The listing builds one solid part. Answer for the finished solid, in the listing's coordinates (mm). Face numbers are marked on the shaded views. A direction names the side the tool comes from. Round coordinates to 2 decimals unless told otherwise and drop trailing zeros. Loops run counter-clockwise (first coordinate to the right, second up) from the corner with the lowest first, then second, coordinate; pieces in that order, holes last. Notation, with made-up numbers: (5.5, 64) -> (43.5, 64) arc R17 cw to (43.5, 78) -> close; hole circle Ø2 at (-12, -19.75). An arc over 180 degrees is marked (long way). One line per question, with ' | ' between items.
from build123d import *

# Parameters (mm, degrees)
F0_W     = 50.8
F0_H     = 50.8
F1_DEPTH = 7.62
F2_T     = -1.27
F3_R     = 1.27
F4_DEPTH = 25.4


with BuildPart() as f1:
    # F0 (on Top) → F1 (new body)
    with BuildSketch(Plane.XY):
        with Locations((25.4, 25.4)):
            Rectangle(F0_W, F0_H)
    extrude(amount=F1_DEPTH)

    # F2
    f2_openings = [f1.faces().sort_by_distance(p)[0] for p in [
        (25.4, 25.4, 7.62),
    ]]
    offset(amount=F2_T, openings=f2_openings)

    # F3 (on face) → F4 (cut)
    with BuildSketch(Plane.XY.offset(1.27)):
        with Locations((3.81, 18.601548)):
            Circle(F3_R)
    extrude(amount=-F4_DEPTH, mode=Mode.SUBTRACT)


solid = f1.part
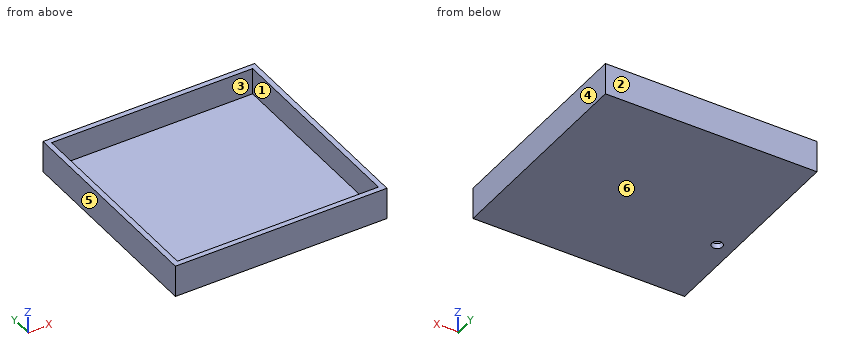
Q1. A cutting plane is placed at C-C on y = 45. Give the vertices of the cut face in (x, z).
Numbers:
outline: (0, 0) -> (50.8, 0) -> (50.8, 7.62) -> (49.53, 7.62) -> (49.53, 1.27) -> (1.27, 1.27) -> (1.27, 7.62) -> (0, 7.62) -> close
Q2. A cutting plane is placed at B-B on z = 6.75. Give the vertices of the cut face in (x, y).
Numbers:
outline: (0, 0) -> (50.8, 0) -> (50.8, 50.8) -> (0, 50.8) -> close; hole (1.27, 1.27) -> (49.53, 1.27) -> (49.53, 49.53) -> (1.27, 49.53) -> close
Q3. For the marked faces 1 and 2, determine the directions among +Z, -Z, +X, -X, +Y, -Y from which every point of the face is accessible in a straight line to the end or side of a thin tool.
Numbers:
face 1: +Z | face 2: +Z, -Z, +X, -X, +Y
Q4. Given pin 1 Ø6 at (x, y) = (26, 25) entering from +Z; pin 2 Ø3 at (x, z) = (29, 5) entering from -Y, each flat-ended and moving along its own axis, determine where each tip first touches the part or whether it passes through.
Numbers:
pin 1: z = 1.27 | pin 2: y = 0
Q5. For a pull along X with two mould halves and no side action, classify the marked faces 3, 4, 5 and 6 as pulls with the +X half, pulls with the -X half, needs draft (parallel to the pull), parting line crosses it, or undercut.
Numbers:
face 3: undercut | face 4: pulls with the +X half | face 5: pulls with the -X half | face 6: needs draft
Q6. A cutting plane is placed at A-A on x = 3.81. Give the vertices of the cut face in (y, z).
Numbers:
outline: (0, 0) -> (17.33, 0) -> (17.33, 1.27) -> (1.27, 1.27) -> (1.27, 7.62) -> (0, 7.62) -> close; (19.87, 0) -> (50.8, 0) -> (50.8, 7.62) -> (49.53, 7.62) -> (49.53, 1.27) -> (19.87, 1.27) -> close
Q7. Find the intervals of material crossed by line 1 (X direction, y = 25, z = 4.25); line 2 (Y direction, x = 3.81, z = 0.5), in increasing order. Write a range as from..to.
Numbers:
line 1: 0..1.27, 49.53..50.8 | line 2: 0..17.33, 19.87..50.8
